For this review, take the finished solid that the model builds, in its own axes (mm). Round coordinates to 2 decimals unless told otherwise and drop trailing zeros. Write each loop counter-clockwise with the first axis right and the second up, starting at its lowest first coordinate (ties: lowest second). Pieces come first, ordered by that corner, then holes. Notation, with made-up numbers: (74.5, 17.25) -> (115.5, 17.25) arc R19 cw to (115.5, 35.25) -> close; hole circle Ø7 at (-9.5, -29.5). An arc over 180 degrees is marked (long way). Write each question's results on one line, items separated by ' | '. Start each with the question number.
Item 1: Add section C-C (x = -17). State the section outline as (y, z) points, plus the area to 3 significant figures.
Item 2: Add section D-D (z = -16). State the section outline as (x, y) points, plus the area to 3 significant figures.
Item 3: Add section B-B (z = 0). State the section outline as (x, y) points.
Item 4: Clearance check with flat-ended pins moving along their axes: pin 1 (1 mm diameter, centred on x = -2, y = 7.5, fed in from +Z); pin 2 (6 mm diameter, centred on y = 8.5, z = 13, fed in from +X); pin 3 (3 mm diameter, centred on x = 16.5, y = 1.5, fed in from +Z). State where each tip first meets the part, or that it passes through.
Item 5: Add section A-A (x = 0). State the section outline as (y, z) points.
Item 6: To check wall thickness, follow line 1 along X through (y, z) = (6, 16); line 2 along X through (y, z) = (2, 0); line 3 along X through (y, z) = (5, 32). State the ranges of each line that lie inside material, in increasing order.
Item 7: The part is to be moulded in two halves that separate along X. For faces 1 (the cylindrical face through (-14.17, 5.07, 34.18)), 2 (the cylindrical face through (-26.36, 5.07, -5.85)), 3 (the flat face through (-27.2, 0, -0.2)), say which applies: +X half, -X half, draft (parallel to the pull), parting line (faces both ways), or undercut.
from build123d import *

# Parameters (mm, degrees)
SKETCH1_R           = 45
BOSS_EXTRUDE1_DEPTH = 10
SKETCH2_R           = 45
SKETCH2_R_2         = 37
SKETCH2_R_3         = 27
CUT_EXTRUDE1_DEPTH  = 10
SKETCH3_R           = 2
CUT_EXTRUDE2_DEPTH  = 10


with BuildPart() as part:
    # Sketch1 → Boss-Extrude1 (new body)
    with BuildSketch(Plane(origin=(0, 0, 0), x_dir=(1, 0, 0), z_dir=(0, 1, 0))):
        with Locations(Location((0, 0, 0), (0, 0, 270))):
            Circle(SKETCH1_R)
    extrude(amount=BOSS_EXTRUDE1_DEPTH)

    # Sketch2 → Cut-Extrude1 (cut)
    with BuildSketch(Plane(origin=(0, 10, 0), x_dir=(1, 0, 0), z_dir=(0, 1, 0))):
        Circle(SKETCH2_R)
        with Locations(Location((0, 0, 0), (0, 0, 270))):
            Circle(SKETCH2_R_2, mode=Mode.SUBTRACT)
        with Locations(Location((0, 0, 0), (0, 0, 270))):
            Circle(SKETCH2_R_3)
    extrude(amount=-CUT_EXTRUDE1_DEPTH, mode=Mode.SUBTRACT)

    # Sketch3 → Cut-Extrude2 (cut)
    with BuildSketch(Plane(origin=(0, 10, 0), x_dir=(1, 0, 0), z_dir=(0, 1, 0))):
        with Locations(Location((0, 32, 0), (0, 0, 270))):
            Circle(SKETCH3_R)
        with Locations(Location((27.712812921, 16, 0), (0, 0, 270))):
            Circle(SKETCH3_R)
        with Locations(Location((27.712812921, -16, 0), (0, 0, 270))):
            Circle(SKETCH3_R)
        with Locations(Location((0, -32, 0), (0, 0, 270))):
            Circle(SKETCH3_R)
        with Locations(Location((-27.712812921, -16, 0), (0, 0, 270))):
            Circle(SKETCH3_R)
        with Locations(Location((-27.712812921, 16, 0), (0, 0, 270))):
            Circle(SKETCH3_R)
    extrude(amount=-CUT_EXTRUDE2_DEPTH, mode=Mode.SUBTRACT)


solid = part.part
Responses:
1) outline: (0, -32.86) -> (10, -32.86) -> (10, -20.98) -> (0, -20.98) -> close; (0, 20.98) -> (10, 20.98) -> (10, 32.86) -> (0, 32.86) -> close | area: 238 mm^2
2) outline: (-33.36, 0) -> (-29.71, 0) -> (-29.71, 10) -> (-33.36, 10) -> close; (-25.71, 0) -> (-21.75, 0) -> (-21.75, 10) -> (-25.71, 10) -> close; (21.75, 0) -> (25.71, 0) -> (25.71, 10) -> (21.75, 10) -> close; (29.71, 0) -> (33.36, 0) -> (33.36, 10) -> (29.71, 10) -> close | area: 152 mm^2
3) outline: (-37, 0) -> (-27, 0) -> (-27, 10) -> (-37, 10) -> close; (27, 0) -> (37, 0) -> (37, 10) -> (27, 10) -> close
4) pin 1: stops at z = 36.97 | pin 2: stops at x = 35.62 | pin 3: stops at z = 33.82
5) outline: (0, -37) -> (10, -37) -> (10, -34) -> (0, -34) -> close; (0, -30) -> (10, -30) -> (10, -27) -> (0, -27) -> close; (0, 27) -> (10, 27) -> (10, 30) -> (0, 30) -> close; (0, 34) -> (10, 34) -> (10, 37) -> (0, 37) -> close
6) line 1: x = -33.36 to -29.71, -25.71 to -21.75, 21.75 to 25.71, 29.71 to 33.36 | line 2: x = -37 to -27, 27 to 37 | line 3: x = -18.57 to -2, 2 to 18.57
7) face 1: parting line | face 2: undercut | face 3: draft
